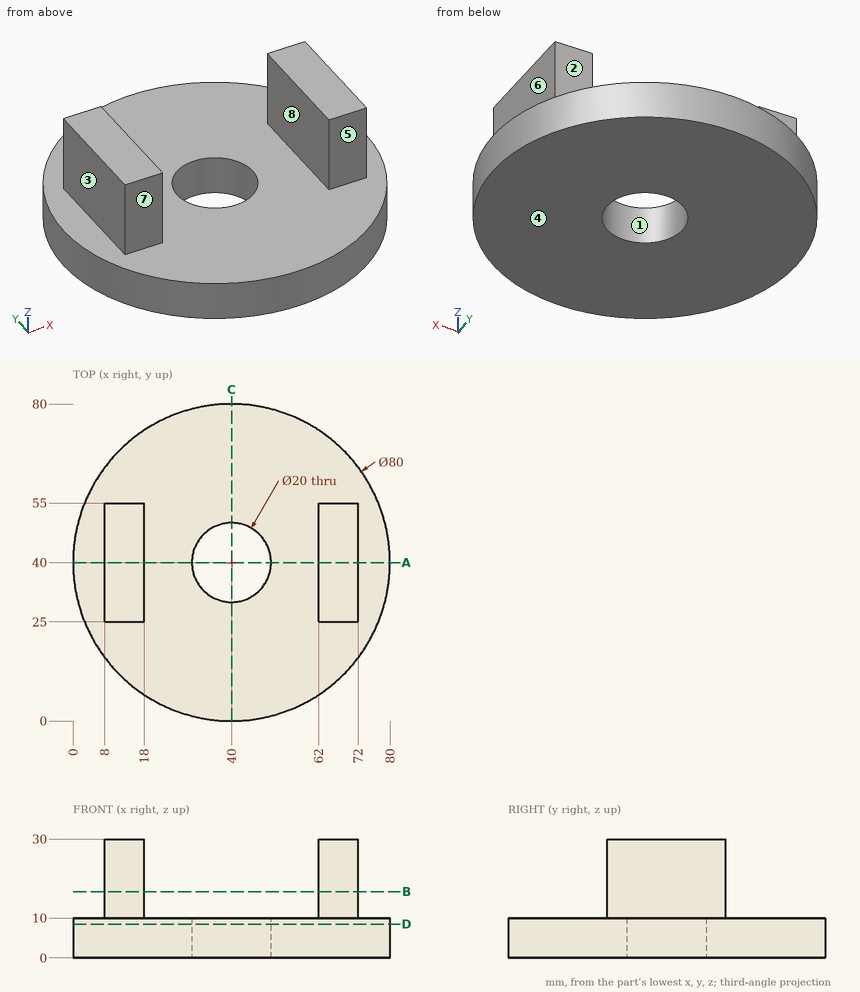
Geometry: see drawing. Coordinates: mm, zero at the bounding-box minimum. A direction names the side the tool comes from. Round coordinates to 2 decimals unless told otherwise and drop trailing zeros. Loops run counter-clockwise (first coordinate to the right, second up) from the corner with the lowest first, then second, coordinate; pieces in that order, holes last. Notation, with made-up numbers: (17.25, 64.5) -> (73.25, 64.5) arc R21 ccw to (73.25, 81.5) -> close; hole circle Ø7 at (57.25, 12.25). An arc over 180 degrees is marked (long way). Write each question's results on one line, items separated by ' | '.
1. Section A-A (y = 40). Return loops of the section in (x, z).
Geometry results:
outline: (0, 0) -> (30, 0) -> (30, 10) -> (18, 10) -> (18, 30) -> (8, 30) -> (8, 10) -> (0, 10) -> close; (50, 0) -> (80, 0) -> (80, 10) -> (72, 10) -> (72, 30) -> (62, 30) -> (62, 10) -> (50, 10) -> close
2. Ray query, line 1 (Y direction, x = 40, z = 3); line 2 (Z direction, x = 55, y = 36.5); line 3 (X direction, y = 31.5, z = 23). Return the intervals inside material, ascending. Write a range as from..to.
Geometry results:
line 1: 0..30, 50..80 | line 2: 0..10 | line 3: 8..18, 62..72
3. First-contact query: P1, Ø6, axis at x = 10, z = 12.5, coming from the +Y side; P2, Ø11, axis at x = 65.5, z = 23, coming from the +Y side; P3, Ø10, axis at y = 42.5, z = 25, coming from the -X side. Flat tips, straight axial feed; report the tip coordinate or a pass-through.
Geometry results:
P1: y = 68.23 | P2: y = 55 | P3: x = 8
4. Mould query, pull axis X, two halves, no side actions, for the marked faces 6, 7 and 8. Classes: +X half, -X half, draft (parallel to the pull), parting line (faces both ways), or undercut.
Geometry results:
face 6: +X half | face 7: draft | face 8: undercut
5. Set-up query: the marked faces 1, 2, 3, 4 and 5. Return all of +Z, -Z, +X, -X, +Y, -Y with unobstructed straight access to the full face (end or side cutting, diameter ignored); none if empty.
Geometry results:
face 1: +Z, -Z | face 2: +Z, +X, -X, +Y | face 3: +Z, -X, +Y, -Y | face 4: -Z, +X, -X, +Y, -Y | face 5: +Z, +X, -X, -Y
6. Section D-D (z = 8.5). Return loops of the section in (x, y), and give its area (3 significant figures).
Geometry results:
outline: circle Ø80 at (40, 40); hole circle Ø20 at (40, 40) | area: 4,710 mm2
7. Section B-B (z = 16.75). Return loops of the section in (x, y), and give its area (3 significant figures).
Geometry results:
outline: (8, 25) -> (18, 25) -> (18, 55) -> (8, 55) -> close; (62, 25) -> (72, 25) -> (72, 55) -> (62, 55) -> close | area: 600 mm2
8. Section C-C (x = 40). Return loops of the section in (y, z), and give its area (3 significant figures).
Geometry results:
outline: (0, 0) -> (30, 0) -> (30, 10) -> (0, 10) -> close; (50, 0) -> (80, 0) -> (80, 10) -> (50, 10) -> close | area: 600 mm2
